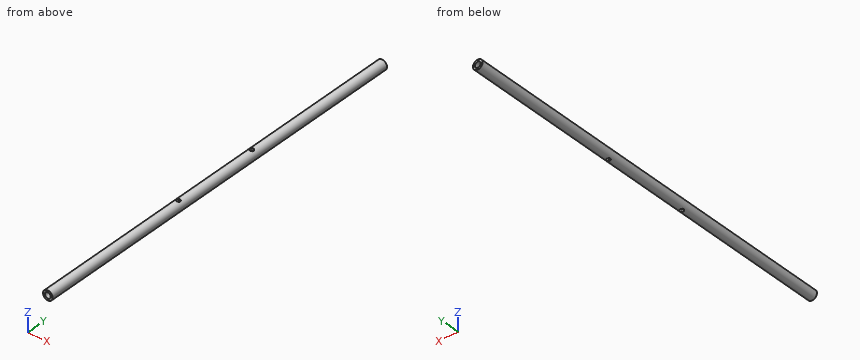
Autodesk Inventor part; units mm, degrees
ref_plane "YZ Plane" through (0, 0, 0) normal (1, 0, 0) x (0, 1, 0)
ref_plane "XZ Plane" through (0, 0, 0) normal (0, 1, 0) x (-1, 0, 0)
ref_plane "XY Plane" through (0, 0, 0) normal (0, 0, 1) x (1, 0, 0)
sketch "Skizze1" plane through (0, 0, 0) normal (0, 1, 0) x (-1, 0, 0)
  circle A0 centre (0, 0) radius 5
  circle A1 centre (0, 0) radius 3
  dimension "d0" = 2
  dimension "d2" = 10
  dimension "d20" = 6
extrude "Extrusion1" add sketch "Skizze1" along normal mid plane 410
ref_plane "Arbeitsebene2" through (0, 0, -5) normal (0, 0, 1) x (1, 0, 0)
ref_plane "Arbeitsebene1" through (-8, 108.509, 24.4581) normal (0, 0, 1) x (0, -1, 0)
sketch "Skizze3" plane through (0, 0, -5) normal (0, 0, 1) x (1, 0, 0)
  line L0 (0, 0) -> (0, 160.2649) construction
  point P0 (0, 0)
  point P1 (0, 80.1325)
  point P2 (0, 45)
  point P3 (0, -45)
  dimension "d8" = 45
  dimension "d10" = 45
hole "Bohrung1" at (0, 45, -5) at (0, -45, -5) direction (0, 0, 1) diameter 4 end through all
ref_plane "Arbeitsebene4" through (0, 0, 5) normal (0, 0, 1) x (1, 0, 0)
thread "Gewinde1"
thread "Gewinde2"
properties part number "Zwischenstange" material "Aluminium"
Design review of the part built by this model. Coordinates are the model's own, in mm. Round coordinates to 2 decimals unless told otherwise and drop trailing zeros. Write each loop counter-clockwise with the first axis right and the second up, starting at its lowest first coordinate (ties: lowest second). Pieces come first, ordered by that corner, then holes. Notation, with made-up numbers: (-13.75, 16) -> (-1.75, 16) arc R13 cw to (-1.75, 31) -> close; hole circle Ø5 at (-3.5, 65.5). An arc over 180 degrees is marked (long way). One line per item, written item: value. Start each with the question number.
Q1. Add section A-A (z = 0). Give the boundary of the cut face in (x, y), then the cut area to 3 significant figures.
Q2. Add section B-B (x = 0). Give the boundary of the cut face in (y, z).
Q3. To check wall thickness, follow probe 1 along Y at (x, z) = (0, 4.2); probe 2 along X at (y, z) = (-45, -3.95); probe 3 along Z at (x, y) = (-0.25, -125.5). State the ranges of each line that lie inside material, in increasing order.
Q4. Add section C-C (y = 138.5). Give the boundary of the cut face in (x, z), then the cut area to 3 significant figures.
Response:
1. outline: (-5, -205) -> (-3, -205) -> (-3, 205) -> (-5, 205) -> close; (3, -205) -> (5, -205) -> (5, 205) -> (3, 205) -> close
1. area: 1,640 mm^2
2. outline: (-205, -5) -> (-47, -5) -> (-47, -3) -> (-205, -3) -> close; (-205, 3) -> (-47, 3) -> (-47, 5) -> (-205, 5) -> close; (-43, -5) -> (43, -5) -> (43, -3) -> (-43, -3) -> close; (-43, 3) -> (43, 3) -> (43, 5) -> (-43, 5) -> close; (47, -5) -> (205, -5) -> (205, -3) -> (47, -3) -> close; (47, 3) -> (205, 3) -> (205, 5) -> (47, 5) -> close
3. probe 1: y = -205 to -47, -43 to 43, 47 to 205
3. probe 2: x = -3.07 to -2, 2 to 3.07
3. probe 3: z = -4.99 to -2.99, 2.99 to 4.99
4. outline: circle Ø10 at (0, 0); hole circle Ø6 at (0, 0)
4. area: 50.3 mm^2
